Design review of the part shown in the three views and the two pictorial views. Dimensions are in mm from the part's minimum x, y and z. A direction names the side the tool comes from. Coordinates: 2 decimals unless noted, no trailing zeros. Loops run counter-clockwise (first coordinate to the right, second up) from the corner with the lowest first, then second, coordinate; pieces in that order, holes last.
Q1. Add section D-D on x = 11.75. Give the boundary of the cut face in (y, z), and give its area (3 significant figures).
Q2. Draft analysis for pull direction X (two halves, no side actions). For the marked faces 4, 5 and 6, state which applies: released by +X, released by -X, zero draft, split by the parting line, or undercut.
Q3. Add section A-A on z = 5. Give the boundary of the cut face in (x, y).
Q4. Machinability: for the marked faces 1, 2 and 3, which of the approach directions +Z, -Z, +X, -X, +Y, -Y give a long, thin tool a straight path to every point of the face, cutting with its end or side? Answer none if there is none.
Q5. Add section C-C on y = 25. Give the boundary of the cut face in (x, z).
Q6. Wall thickness on probe 1 along Y at (x, z) = (18.75, 11.5); probe 2 along Z at (x, y) = (22.5, 0.95); probe 3 along Y at (x, z) = (21.25, 1.5): over which ranges is each line inside the solid? List them lowest first.
Q7. For P1, Ø5, axis at x = 22, y = 8, coming from the -Z side; P2, Ø4, axis at x = 7.5, z = 5, coming from the +Y side, all flat-tipped, find the tip position at first contact; note any pin that passes through.
Q8. Add section B-B on x = 7.5. Give the boundary of the cut face in (y, z), and give its area (3 significant figures).
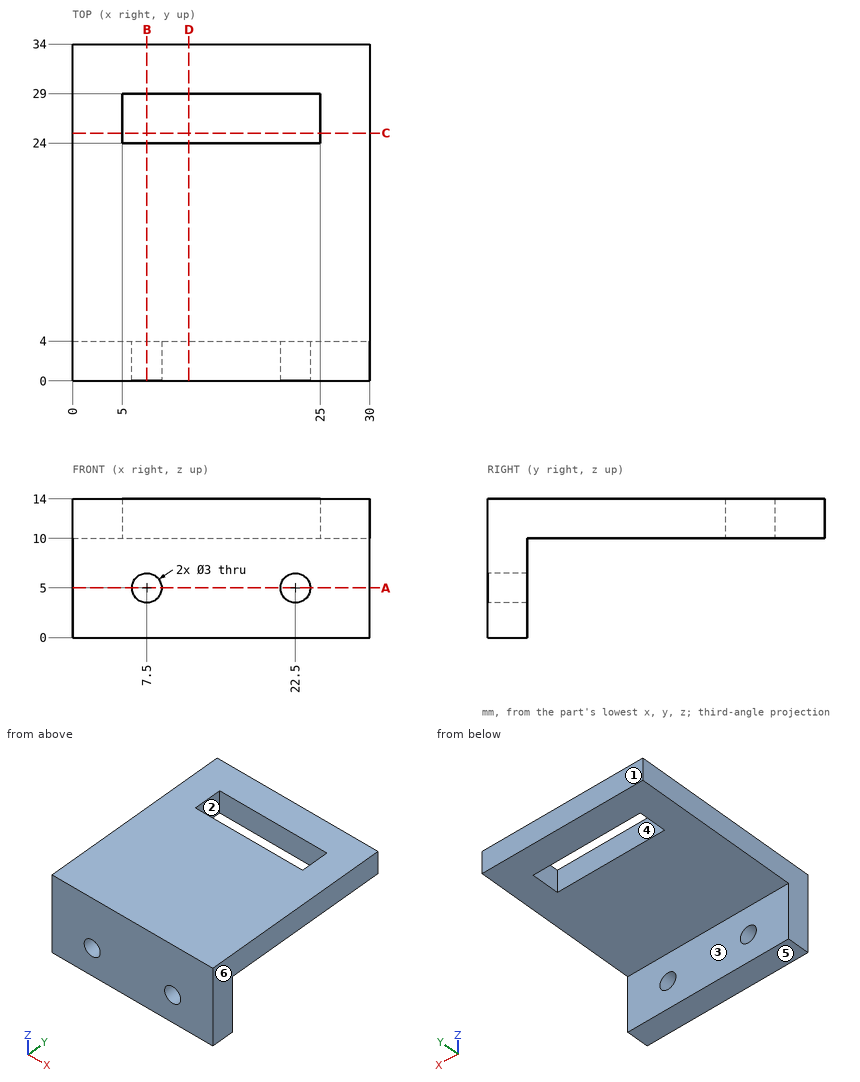
Entries:
1. outline: (0, 0) - (4, 0) - (4, 10) - (24, 10) - (24, 14) - (0, 14) - close; (29, 10) - (34, 10) - (34, 14) - (29, 14) - close
1. area: 156 mm2
2. face 4: undercut
2. face 5: zero draft
2. face 6: released by +X
3. outline: (0, 0) - (6, 0) - (6, 4) - (0, 4) - close; (9, 0) - (21, 0) - (21, 4) - (9, 4) - close; (24, 0) - (30, 0) - (30, 4) - (24, 4) - close
4. face 1: +Z, -Z, +X, -X, +Y
4. face 2: +Z, -Z
4. face 3: -Z, +X, -X, +Y
5. outline: (0, 10) - (5, 10) - (5, 14) - (0, 14) - close; (25, 10) - (30, 10) - (30, 14) - (25, 14) - close
6. probe 1: y = 0 to 24, 29 to 34
6. probe 2: z = 0 to 3.5, 6.5 to 14
6. probe 3: y = 0 to 4
7. P1: stops at z = 10
7. P2: stops at y = 4
8. outline: (0, 0) - (4, 0) - (4, 3.5) - (0, 3.5) - close; (0, 6.5) - (4, 6.5) - (4, 10) - (24, 10) - (24, 14) - (0, 14) - close; (29, 10) - (34, 10) - (34, 14) - (29, 14) - close
8. area: 144 mm2
